Solid Edge part; units mm, degrees
sketch "Sketch1" plane through (0, 0, 0) normal (1, 0, 0) x (0, 1, 0)
  line L0 (0, -10) -> (6, -10)
  line L1 (6, -10) -> (14.6603, -5)
  line L2 (14.6603, 5) -> (14.6603, -5)
  line L3 (6, 10) -> (14.6603, 5)
  line L4 (0, 10) -> (6, 10)
  line L5 (0, 4.5) -> (0, 10)
  line L6 (2, 4.5) -> (0, 4.5)
  line L7 (2, 2.5) -> (2, 4.5)
  line L8 (0, 2.5) -> (2, 2.5)
  line L9 (0, 0) -> (0, 2.5)
  line L10 (0, 0) -> (0, -2.5)
  line L11 (0, -2.5) -> (2, -2.5)
  line L12 (2, -2.5) -> (2, -4.5)
  line L13 (2, -4.5) -> (0, -4.5)
  line L14 (0, -4.5) -> (0, -10)
  dimension "D1" = 6
  dimension "D2" = 2
  dimension "D3" = 2
  dimension "D4" = 2
extrude "Ajout_matière_1" add sketch "Sketch1" along normal mid plane 8
hole "Perçage_1" at (4, 3, 7) direction (-1, 0, 0) diameter 3 end up to next
hole "Hole1" at (4, 3, -7) direction (-1, 0, 0) diameter 3 end up to next
hole "Perçage_3" at (4, 3, 0) direction (-1, 0, 0) diameter 2.621 end up to next
hole "Perçage_4" at (4, 10.3301, 0) direction (-1, 0, 0) diameter 4.134 end up to next
chamfer "Chanfrein_1" distance 0.5 angle 45 10 edges at (-4, 14.6603, 0) (4, 14.6603, 0) (0, 14.6603, 5) (0, 14.6603, -5) (-4, 10.3301, 7.5) (4, 10.3301, 7.5) (-4, 10.3301, -7.5) (4, 10.3301, -7.5) (0, 6, 10) (0, 6, -10)
properties material "Aluminium AU4G, 2024_T4"
Input: part model. Units: mm. Frame: model coordinates. A direction names the side the tool comes from. Coordinates: 2 decimals unless noted, no trailing zeros. Loops run counter-clockwise (first coordinate to the right, second up) from the corner with the lowest first, then second, coordinate; pieces in that order, holes last. Notation, with made-up numbers: (78.5, 31) -> (132.5, 31) arc R17 cw to (132.5, 59) -> close; hole circle Ø9 at (38, 18.25). An arc over 180 degrees is marked (long way). Use a Markdown table: item, result.
1) Cut plane D-D (z = -7.75). Return the cut outline in (x, y), then the cut area to 3 significant figures.
Results found:
| item | result |
|---|---|
| outline | (-4, 0) -> (4, 0) -> (4, 1.7) -> (-4, 1.7) -> close; (-4, 4.3) -> (4, 4.3) -> (4, 8.9) -> (3.5, 9.9) -> (-3.5, 9.9) -> (-4, 8.9) -> close |
| area | 57.9 mm2 |
2) Access query for faces 4 (the flat face through (-0.05, 10.28, -7.53)), 5 (the flat face through (0, 1, 2.5)). Directions: +Z, -Z, +X, -X, +Y, -Y. A direction counts if a zero-diameter tool reaches every point of the face in a straight line with its end or side. Return the directions, or none.
Results found:
| item | result |
|---|---|
| face 4 | -Z, +X, -X, +Y |
| face 5 | +X, -X, -Y |
3) Cut plane A-A (z = 0). Return the cut outline in (x, y).
Results found:
| item | result |
|---|---|
| outline | (-4, 0) -> (4, 0) -> (4, 1.69) -> (-4, 1.69) -> close; (-4, 4.31) -> (4, 4.31) -> (4, 8.26) -> (-4, 8.26) -> close; (-4, 12.4) -> (4, 12.4) -> (4, 14.16) -> (3.5, 14.66) -> (-3.5, 14.66) -> (-4, 14.16) -> close |
4) Cut plane C-C (y = 1.25). Return the cut outline in (x, z), then the cut area to 3 significant figures.
Results found:
| item | result |
|---|---|
| outline | (-4, -10) -> (4, -10) -> (4, -4.5) -> (-4, -4.5) -> close; (-4, -2.5) -> (4, -2.5) -> (4, 2.5) -> (-4, 2.5) -> close; (-4, 4.5) -> (4, 4.5) -> (4, 10) -> (-4, 10) -> close |
| area | 128 mm2 |
5) Cut plane B-B (y = 3). Return the cut outline in (x, z).
Results found:
| item | result |
|---|---|
| outline | (-4, -10) -> (4, -10) -> (4, -8.5) -> (-4, -8.5) -> close; (-4, -5.5) -> (4, -5.5) -> (4, -1.31) -> (-4, -1.31) -> close; (-4, 1.31) -> (4, 1.31) -> (4, 5.5) -> (-4, 5.5) -> close; (-4, 8.5) -> (4, 8.5) -> (4, 10) -> (-4, 10) -> close |
6) Contact query for flat-ended pins moving along their axis: pin 1 (1.8 mm diameter, centred on y = 3, z = -7, fed in from -X); pin 2 (1.6 mm diameter, centred on x = -1.5, z = -3.5, fed in from -Y). Output: stop coordinate, or through.
Results found:
| item | result |
|---|---|
| pin 1 | passes through |
| pin 2 | stops at y = 2 |
7) Pull-direction query (Z, two-part tool) for faces 1 (the flat face through (0, 2, -3)), 2 (the flat face through (0, 0, 7)), 3 (the flat face through (-0.052, 5.973, 9.873)); classes: released by +Z, released by -Z, zero draft, split by the parting line, or undercut.
Results found:
| item | result |
|---|---|
| face 1 | undercut |
| face 2 | zero draft |
| face 3 | released by +Z |
8) Material intervals for line 1 along Z through (x, y) = (1, 3); line 2 along Z through (x, y) = (2, 1.25); line 3 along Y through (x, z) = (1.25, 0), sorted ascending. Write a range as from..to.
Results found:
| item | result |
|---|---|
| line 1 | z = -10..-8.5, -5.5..-1.31, 1.31..5.5, 8.5..10 |
| line 2 | z = -10..-4.5, -2.5..2.5, 4.5..10 |
| line 3 | y = 0..1.69, 4.31..8.26, 12.4..14.66 |
